Geometry: see drawing. Coordinates: mm, zero at the bounding-box minimum. A direction names the side the tool comes from. Coordinates: 2 decimals unless noted, no trailing zeros. Order: outer loops, then holes, each group sorted by start corner. A loop starts at its lowest first (then second) coordinate and runs counter-clockwise, first axis right, second up. Notation, with made-up numbers: (81, -16) -> (96, -16) arc R21 ccw to (96, 8) -> close; hole circle Ø4 at (67.5, 43.25). An arc over 180 degrees is marked (long way). Use one line per item in the form item = value.
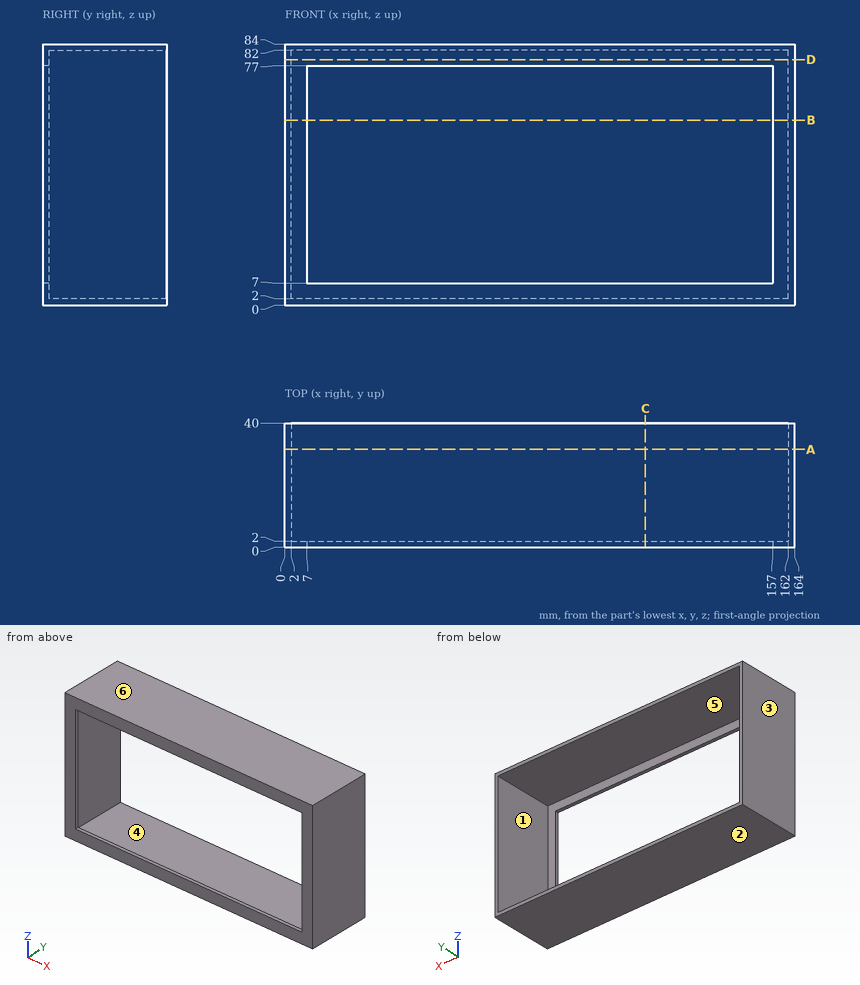
1) Section D-D, the plane z = 79. Output: boundary loops of the cut face in (x, y).
Results found:
outline = (0, 0) -> (164, 0) -> (164, 40) -> (162, 40) -> (162, 2) -> (2, 2) -> (2, 40) -> (0, 40) -> close
2) Pull-direction query (Z, two-part tool) for the marked faces 3, 4, 5 and 6; classes: released by +Z, released by -Z, zero draft, split by the parting line, or undercut.
Results found:
face_3 = zero draft
face_4 = undercut
face_5 = undercut
face_6 = released by +Z
3) Section C-C, the plane x = 116. Output: boundary loops of the cut face in (y, z), and give its area (3 significant figures).
Results found:
outline = (0, 0) -> (40, 0) -> (40, 2) -> (2, 2) -> (2, 7) -> (0, 7) -> close; (0, 77) -> (2, 77) -> (2, 82) -> (40, 82) -> (40, 84) -> (0, 84) -> close
area = 180 mm2
4) Section B-B, the plane z = 59.5. Output: boundary loops of the cut face in (x, y), and give its area (3 significant figures).
Results found:
outline = (0, 0) -> (7, 0) -> (7, 2) -> (2, 2) -> (2, 40) -> (0, 40) -> close; (157, 0) -> (164, 0) -> (164, 40) -> (162, 40) -> (162, 2) -> (157, 2) -> close
area = 180 mm2
5) Section A-A, the plane y = 31.5. Output: boundary loops of the cut face in (x, z), and give its area (3 significant figures).
Results found:
outline = (0, 0) -> (164, 0) -> (164, 84) -> (0, 84) -> close; hole (2, 2) -> (162, 2) -> (162, 82) -> (2, 82) -> close
area = 976 mm2
6) Access query for the marked faces 1 and 2. Directions: +Z, -Z, +X, -X, +Y, -Y. A direction counts if a zero-diameter tool reaches every point of the face in a straight line with its end or side. Return the directions, or none.
Results found:
face_1 = +Y
face_2 = -Z, +X, -X, +Y, -Y
7) Material intervals for probe 1 along X at (y, z) = (11.5, 26.5); probe 2 along Z at (x, y) = (112, 28.5), sorted ascending. Write a range as from..to.
Results found:
probe_1 = 0..2, 162..164
probe_2 = 0..2, 82..84
